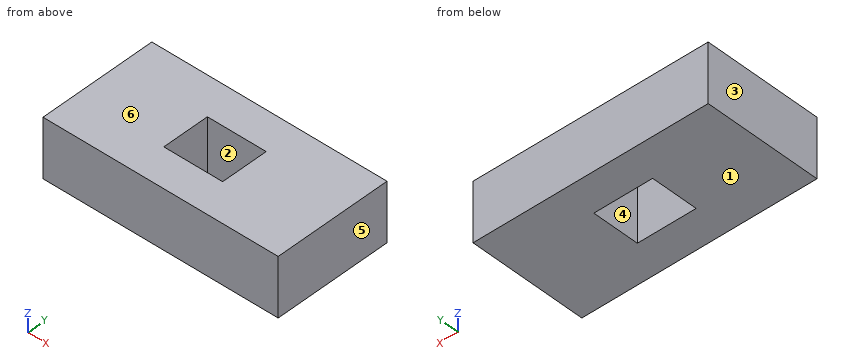
```python
from build123d import *

# Parameters (mm, degrees)
RECTANGLESKETCH_W   = 40
RECTANGLESKETCH_H   = 20
BLINDBOSS_DEPTH     = 10
CUTSKETCH_W         = 10
CUTSKETCH_H         = 8
THROUGHALLCUT_DEPTH = 46.82575695


with BuildPart() as part:
    # RectangleSketch → BlindBoss (new body)
    with BuildSketch(Plane.XY):
        with Locations((20, 10)):
            Rectangle(RECTANGLESKETCH_W, RECTANGLESKETCH_H)
    extrude(amount=BLINDBOSS_DEPTH)

    # CutSketch → ThroughAllCut (cut, through all)
    with BuildSketch(Plane.XY.offset(10)):
        with Locations((20, 10)):
            Rectangle(CUTSKETCH_W, CUTSKETCH_H)
    extrude(amount=-THROUGHALLCUT_DEPTH, mode=Mode.SUBTRACT)


solid = part.part
```
The model under review builds one solid part; all positions refer to its coordinate system, in mm. Face numbers are marked on the shaded views. A direction names the side the tool comes from. Give positions to 0.01 mm unless a question says otherwise; leave off trailing zeros. Loops run counter-clockwise (first coordinate to the right, second up) from the corner with the lowest first, then second, coordinate; pieces in that order, holes last. Notation, with made-up numbers: (3.25, -34.5) - (51.25, -34.5) arc R24 ccw to (51.25, -9.5) - close; hole circle Ø5 at (38, 16). An arc over 180 degrees is marked (long way). Answer as a JSON object with one key per item and string values.
Q1. Add section C-C on z = 6.75. State the section outline as (x, y) points, plus the area to 3 significant figures.
Worked out:
{"outline": "(0, 0) - (40, 0) - (40, 20) - (0, 20) - close; hole (15, 6) - (25, 6) - (25, 14) - (15, 14) - close", "area": "720 mm^2"}
Q2. To check wall thickness, follow line 1 along X through (y, z) = (13, 4); line 2 along Y through (x, z) = (16.5, 2.5). State the ranges of each line that lie inside material, in increasing order.
Worked out:
{"line 1": "x = 0 to 15, 25 to 40", "line 2": "y = 0 to 6, 14 to 20"}
Q3. Mouldability with a two-part tool opening along X and no side actions: class the marked faces 3, 4, 5 and 6 as +X half, -X half, draft (parallel to the pull), parting line (faces both ways), or undercut.
Worked out:
{"face 3": "-X half", "face 4": "undercut", "face 5": "+X half", "face 6": "draft"}
Q4. For the marked faces 1 and 2, list the 3-axis set-ups (+Z, -Z, +X, -X, +Y, -Y) from which the entire face can be reached by the end or side of a thin tool; tool diameter is ignored.
Worked out:
{"face 1": "-Z, +X, -X, +Y, -Y", "face 2": "+Z, -Z"}
Q5. Add section B-B on x = 20.5. State the section outline as (y, z) points.
Worked out:
{"outline": "(0, 0) - (6, 0) - (6, 10) - (0, 10) - close; (14, 0) - (20, 0) - (20, 10) - (14, 10) - close"}
Q6. Add section A-A on y = 12. State the section outline as (x, z) points.
Worked out:
{"outline": "(0, 0) - (15, 0) - (15, 10) - (0, 10) - close; (25, 0) - (40, 0) - (40, 10) - (25, 10) - close"}
